Source: CAD feature listing. Evaluate the final solid. Frame: model axes, mm. Give positions to 0.01 mm unless a question says otherwise; leave off trailing zeros. Loops run counter-clockwise (first coordinate to the right, second up) from the corner with the lowest first, then second, coordinate; pieces in that order, holes last.
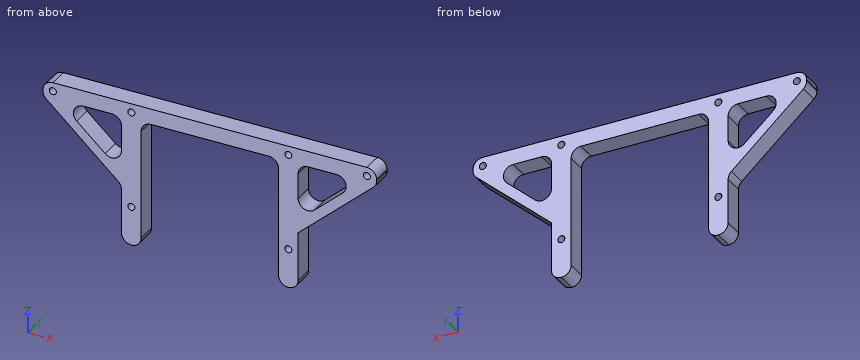
```python
from build123d import *

# Parameters (mm, degrees)
SKETCH2_R           = 2.286
BOSS_EXTRUDE1_DEPTH = 12.7
FILLET1_R           = 6.35


with BuildPart() as part:
    # Sketch2 → Boss-Extrude1 (new body)
    with BuildSketch(Plane(origin=(0, 0, 0), x_dir=(1, 0, 0), z_dir=(0, 1, 0))):
        Polygon((107.95, 0), (-107.95, 0), (-107.95, 10.16), (-57.15, 55.88), (-57.15, 93.98), (-44.45, 93.98), (-44.45, 10.16), (44.45, 10.16), (44.45, 93.98), (57.15, 93.98), (57.15, 55.88), (107.95, 10.16), align=None)
        with Locations(Location((-50.8, 68.58, 0), (0, 0, 270))):
            Circle(SKETCH2_R, mode=Mode.SUBTRACT)
        with Locations(Location((50.8, 68.58, 0), (0, 0, 90))):
            Circle(SKETCH2_R, mode=Mode.SUBTRACT)
        with Locations(Location((-101.6, 5.715, 0), (0, 0, 270))):
            Circle(SKETCH2_R, mode=Mode.SUBTRACT)
        with Locations(Location((-50.8, 5.715, 0), (0, 0, 270))):
            Circle(SKETCH2_R, mode=Mode.SUBTRACT)
        with Locations(Location((101.6, 5.715, 0), (0, 0, 90))):
            Circle(SKETCH2_R, mode=Mode.SUBTRACT)
        with Locations(Location((50.8, 5.715, 0), (0, 0, 90))):
            Circle(SKETCH2_R, mode=Mode.SUBTRACT)
        Polygon((-57.15, 10.16), (-98.457720811, 10.16), (-57.15, 47.33694873), align=None, mode=Mode.SUBTRACT)
        Polygon((57.15, 47.33694873), (57.15, 10.16), (98.457720811, 10.16), align=None, mode=Mode.SUBTRACT)
    extrude(amount=BOSS_EXTRUDE1_DEPTH)

    # Fillet1
    fillet1_edges = [part.edges().sort_by_distance(p)[0] for p in [
        (57.15, 6.35, -93.98),
        (44.45, 6.35, -93.98),
        (-44.45, 6.35, -93.98),
        (-57.15, 6.35, -93.98),
        (-107.95, 6.35, -10.16),
        (-107.95, 6.35, 0),
        (107.95, 6.35, -10.16),
        (107.95, 6.35, 0),
        (98.457720811, 6.35, -10.16),
        (57.15, 6.35, -47.33694873),
        (57.15, 6.35, -10.16),
        (44.45, 6.35, -10.16),
        (-44.45, 6.35, -10.16),
        (-57.15, 6.35, -10.16),
        (-98.457720811, 6.35, -10.16),
        (-57.15, 6.35, -47.33694873),
        (-57.15, 6.35, -55.88),
    ]]
    fillet(fillet1_edges, radius=FILLET1_R - 0.0001)  # a hair under: the kernel refuses the full size


solid = part.part
```
(1) Section C-C, the plane z = -24. Return the cut outline in (x, y), then the cut area to 3 significant figures.
A:
outline: (-92.57, 0) - (-83.08, 0) - (-83.08, 12.7) - (-92.57, 12.7) - close; (-57.15, 0) - (-44.45, 0) - (-44.45, 12.7) - (-57.15, 12.7) - close; (44.45, 0) - (57.15, 0) - (57.15, 12.7) - (44.45, 12.7) - close; (83.08, 0) - (92.57, 0) - (92.57, 12.7) - (83.08, 12.7) - close
area: 564 mm2
(2) Section D-D, the plane y = 4.5. Count the separate pieces of the cut face and the enclosed holes in it, then the cut area to 3 significant figures.
A:
separate pieces: 1
enclosed holes: 8
area: 5,190 mm2
(3) Ray query, line 1 along X through (y, z) = (5.25, -68.58); line 2 along X through (y, z) = (8, -6); line 3 along Z through (x, y) = (50.8, 8). Return the intervals inside material, ascending.
A:
line 1: x = -57.15 to -53.09, -48.51 to -44.45, 44.45 to 48.51, 53.09 to 57.15
line 2: x = -107.94 to -103.87, -99.33 to -53.07, -48.53 to 48.53, 53.07 to 99.33, 103.87 to 107.94
line 3: z = -93.98 to -70.87, -66.29 to -8, -3.43 to 0
(4) Section A-A, the plane z = -63.5. Return the cut outline in (x, y).
A:
outline: (-57.15, 0) - (-44.45, 0) - (-44.45, 12.7) - (-57.15, 12.7) - close; (44.45, 0) - (57.15, 0) - (57.15, 12.7) - (44.45, 12.7) - close
(5) Section B-B, the plane x = -78. Return the cut outline in (y, z) (3 decimals).
A:
outline: (0, -37.115) - (12.7, -37.115) - (12.7, -28.572) - (0, -28.572) - close; (0, -10.16) - (12.7, -10.16) - (12.7, 0) - (0, 0) - close
(6) First-contact query: pin 1 (4 mm diameter, centred on x = 12.5, y = 7.5, fed in from -Z); pin 2 (6 mm diameter, centred on x = -50.8, z = -68.58, fed in from +Y); pin 3 (1.5 mm diameter, centred on y = 11, z = -42, fed in from +X); pin 4 (4 mm diameter, centred on y = 6, z = -76, fed in from -X). Flat tips, straight axial feed; report the tip coordinate or a pass-through.
A:
pin 1: stops at z = -10.16
pin 2: stops at y = 12.7
pin 3: stops at x = 73.41
pin 4: stops at x = -57.15
